Could you check a few things on this model? Use its own coordinates, in mm. Coordinates: 2 decimals unless noted, no trailing zeros. Write each loop counter-clockwise with the first axis right and the second up, starting at its lowest first coordinate (ties: lowest second). Pieces come first, ordered by that corner, then holes. Notation, with made-up numbers: (1.25, -38.5) - (29.25, -38.5) arc R22 ccw to (29.25, -19.5) - close; hole circle Ø2 at (50, -13.75). An arc over 180 degrees is marked (long way). Write item = value, one per line. Start each with the question number.
```python
from build123d import *

# Parameters (mm, degrees)
F1_DEPTH = 50.8


with BuildPart() as f1:
    # F0 (on Front) → F1 (new body)
    with BuildSketch(Plane.XZ):
        with BuildLine():
            Line((-51.3954042884, 6.4779423518), (-61.5453907135, 20.3519611838))
            ThreePointArc((-61.5453907135, 20.3519611838), (-60.8667138024, 18.6005583406), (-60.0787079167, 16.8955477856))
            Line((-60.0787079167, 16.8955477856), (-54.2455671219, 8.922226261))
            ThreePointArc((-54.2455671219, 8.922226261), (-52.8591429812, 7.6550079014), (-51.3954042884, 6.4779423518))
        make_face()
        with BuildLine():
            ThreePointArc((-6.0226364292, 41.4420108727), (-44.0692352638, 57.9743919714), (-61.5453907135, 20.3519611838))
            Line((-61.5453907135, 20.3519611838), (-51.3954042884, 6.4779423518))
            ThreePointArc((-51.3954042884, 6.4779423518), (-25.6375926651, 1.5636092662), (-6.0226364292, 18.9667417762))
            ThreePointArc((-6.0226364292, 18.9667417762), (-8.2795262845, 30.2043763245), (-6.0226364292, 41.4420108727))
        make_face()
        with BuildLine():
            Line((-54.2455671219, 8.922226261), (-60.0787079167, 16.8955477856))
            ThreePointArc((-60.0787079167, 16.8955477856), (-57.8142370593, 13.1083030608), (-55.0137343474, 9.6982832032))
            ThreePointArc((-55.0137343474, 9.6982832032), (-54.6332168762, 9.3067248454), (-54.2455671219, 8.922226261))
        make_face()
        with BuildLine():
            ThreePointArc((49.9324337511, 30.2043763245), (26.557465469, 58.7405564697), (-6.0226364292, 41.4420108727))
            ThreePointArc((-6.0226364292, 41.4420108727), (-4.3721548681, 35.9305871783), (-3.8150285088, 30.2043763245))
            ThreePointArc((-3.8150285088, 30.2043763245), (-4.3721548681, 24.4781654706), (-6.0226364292, 18.9667417762))
            ThreePointArc((-6.0226364292, 18.9667417762), (14.6704111622, 1.7568595144), (40.6273265146, 8.8716899044))
            Line((40.6273265146, 8.8716899044), (49.5864414711, 25.7298732103))
            ThreePointArc((49.5864414711, 25.7298732103), (49.8458067689, 27.9604462466), (49.9324337511, 30.2043763245))
        make_face()
        with BuildLine():
            ThreePointArc((-3.8150285088, 30.2043763245), (-4.3721548681, 35.9305871783), (-6.0226364292, 41.4420108727))
            ThreePointArc((-6.0226364292, 41.4420108727), (-8.2795262845, 30.2043763245), (-6.0226364292, 18.9667417762))
            ThreePointArc((-6.0226364292, 18.9667417762), (-4.3721548681, 24.4781654706), (-3.8150285088, 30.2043763245))
        make_face()
        with BuildLine():
            ThreePointArc((-6.0226364292, 18.9667417762), (-25.6375926651, 1.5636092662), (-51.3954042884, 6.4779423518))
            ThreePointArc((-51.3954042884, 6.4779423518), (-52.8591429812, 7.6550079014), (-54.2455671219, 8.922226261))
            ThreePointArc((-54.2455671219, 8.922226261), (-54.6332168762, 9.3067248454), (-55.0137343474, 9.6982832032))
            Line((-55.0137343474, 9.6982832032), (-14.1391605139, -46.1731813848))
            add(Edge.make_bspline(
                [(-14.1391605139, -46.1731813848), (-11.8439830731, -50.1050845186), (-7.5927454261, -57.3879439304), (4.7284603427, -60.0028426907), (8.5254006183, -51.0662741363), (10.6043620035, -46.1731813848)],
                knots=[0, 0, 0, 0, 0.3467922767, 0.6423452742, 1, 1, 1, 1], degree=3))
            Line((10.6043620035, -46.1731813848), (30.6583169634, -9.8867913974))
            Line((30.6583169634, -9.8867913974), (40.6273265146, 8.8716899044))
            ThreePointArc((40.6273265146, 8.8716899044), (14.6704111622, 1.7568595144), (-6.0226364292, 18.9667417762))
        make_face()
        with BuildLine():
            ThreePointArc((48.2141880079, 20.3519611838), (49.0287968317, 23.0081330988), (49.5864414711, 25.7298732103))
            Line((49.5864414711, 25.7298732103), (40.6273265146, 8.8716899044))
            ThreePointArc((40.6273265146, 8.8716899044), (41.0589651736, 9.2806206), (41.4821603951, 9.6982832032))
            ThreePointArc((41.4821603951, 9.6982832032), (42.2370183544, 10.4877387966), (42.9617238671, 11.3049612832))
            Line((42.9617238671, 11.3049612832), (48.2141880079, 20.3519611838))
        make_face()
        with BuildLine():
            ThreePointArc((41.4821603951, 9.6982832032), (41.0589651736, 9.2806206), (40.6273265146, 8.8716899044))
            Line((40.6273265146, 8.8716899044), (30.6583169634, -9.8867913974))
            Line((30.6583169634, -9.8867913974), (41.4821603951, 9.6982832032))
        make_face()
        with BuildLine():
            ThreePointArc((42.9617238671, 11.3049612832), (45.9977477646, 15.590546245), (48.2141880079, 20.3519611838))
            Line((48.2141880079, 20.3519611838), (42.9617238671, 11.3049612832))
        make_face()
        with BuildLine():
            ThreePointArc((42.9617238671, 11.3049612832), (42.2370183544, 10.4877387966), (41.4821603951, 9.6982832032))
            Line((41.4821603951, 9.6982832032), (30.6583169634, -9.8867913974))
            Line((30.6583169634, -9.8867913974), (42.9617238671, 11.3049612832))
        make_face()
    extrude(amount=F1_DEPTH)


solid = f1.part
```
1) Suppose I cut it at B-B on x = -46. Please give me the cut outline in (y, z).
2) If I drill on probe 1 along X at (y, z) = (-15, 52.5); probe 2 along X at (y, z) = (-4.5, 18); probe 3 along Z at (x, y) = (-12.5, -2.5), over which ranges is the centre line in solid material (lowest first)? Write a range as [from, to].
3) Suppose I cut it at C-C on z = -8.5. Please give me the cut outline in (x, y), plus the area to 3 significant figures.
4) For P1, Ø8, axis at y = -24, z = -14.5, coming from the +X side; P2, Ø1.5, axis at y = -43.5, z = -32, coming from the +X side; P3, Ø2, axis at y = -30.5, z = 19, coming from the +X side (3 decimals), each with a flat end and sliding along its axis, tell me the tip position at first contact or that it passes through.
5) Suppose I cut it at A-A on z = 52.5. Please give me the cut outline in (x, y), plus the area to 3 significant figures.
Reply:
q1.outline = (-50.8, -2.62) - (0, -2.62) - (0, 57.16) - (-50.8, 57.16) - close
q2.probe_1 = [-53.15, -13.89], [2.12, 39.54]
q2.probe_2 = [-60.6, 47.25]
q2.probe_3 = [-48.94, 51.19]
q3.outline = (-41.7, -50.8) - (31.46, -50.8) - (31.46, 0) - (-41.7, 0) - close
q3.area = 3,720 mm^2
q4.P1 = 30.32
q4.P2 = 18.85
q4.P3 = 48.085
q5.outline = (-53.15, -50.8) - (-13.89, -50.8) - (-13.89, 0) - (-53.15, 0) - close; (2.12, -50.8) - (39.54, -50.8) - (39.54, 0) - (2.12, 0) - close
q5.area = 3,900 mm^2
